For this review, use the dimensioned drawing (mm, ordinates from the lowest corner) and the shaded views. Give positions to 0.01 mm unless a question says otherwise; leave off trailing zeros. Write each loop counter-clockwise with the first axis right and the second up, starting at its lowest first coordinate (ties: lowest second). Pieces come first, ordered by that corner, then holes. Notation, with made-up numbers: M -37,72 L -5,72 A31 cw -5,109 Z; hole C 56,66.5 d8. An arc over 180 degrees is marked long. Write each question's results on one line, items separated by ' | '. Start each with the question number.
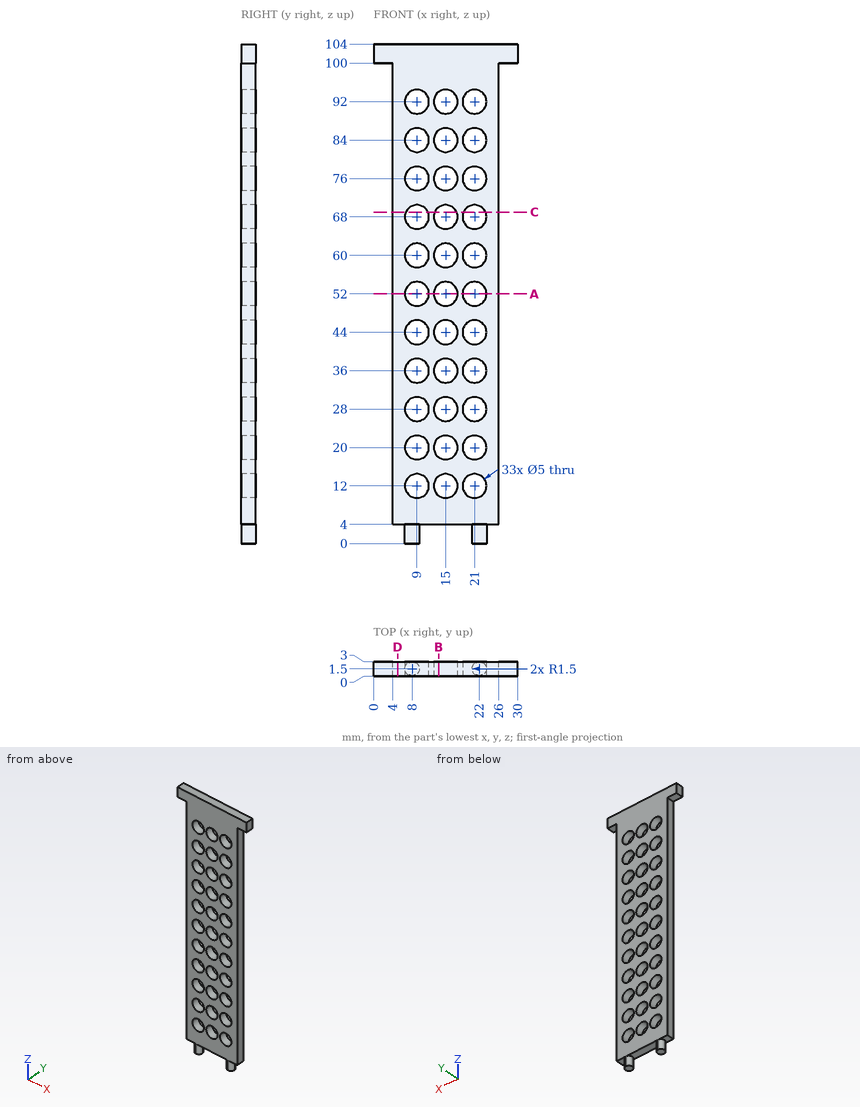
(1) Add section B-B (x = 13.5). Give the number of separate pieces and of enclosed holes in the cut face, then the cut area to 3 significant figures.
(2) Add section D-D (x = 5). State the section outline as (y, z) points.
(3) Wall thickness on L1, parallel to X at y = 2.7, z = 61; L2, parallel to X at y = 2.7, z = 37.5; L3, parallel to Z at x = 4.75, y = 1.8: over which ranges is each line inside the solid? List them lowest first.
(4) Add section C-C (z = 69). State the section outline as (x, y) points, then the cut area to 3 significant figures.
(5) Add section A-A (z = 52). State the section outline as (x, y) points, then the cut area to 3 significant figures.
Calculated:
1) separate pieces: 12 | enclosed holes: 0 | area: 168 mm²
2) outline: M 0,4 L 3,4 L 3,104 L 0,104 Z
3) L1: x = 4 to 6.71, 11.29 to 12.71, 17.29 to 18.71, 23.29 to 26 | L2: x = 4 to 7, 11 to 13, 17 to 19, 23 to 26 | L3: z = 4 to 104
4) outline: M 4,0 L 6.71,0 L 6.71,3 L 4,3 Z; M 11.29,0 L 12.71,0 L 12.71,3 L 11.29,3 Z; M 17.29,0 L 18.71,0 L 18.71,3 L 17.29,3 Z; M 23.29,0 L 26,0 L 26,3 L 23.29,3 Z | area: 24.8 mm²
5) outline: M 4,0 L 6.5,0 L 6.5,3 L 4,3 Z; M 11.5,0 L 12.5,0 L 12.5,3 L 11.5,3 Z; M 17.5,0 L 18.5,0 L 18.5,3 L 17.5,3 Z; M 23.5,0 L 26,0 L 26,3 L 23.5,3 Z | area: 21.0 mm²
